from build123d import *

# Parameters (mm, degrees)
SKETCH1_W           = 19.05
SKETCH1_H           = 19.05
SKETCH1_R           = 4.8895
BOSS_EXTRUDE1_DEPTH = 3.175
SKETCH3_W           = 19.05
SKETCH3_H           = 19.05
SKETCH3_R           = 3.3782
BOSS_EXTRUDE2_DEPTH = 3.175
SKETCH4_W           = 19.05
SKETCH4_H           = 19.05
BOSS_EXTRUDE3_DEPTH = 3.175
FILLET1_R           = 3.175


with BuildPart() as part:
    # Sketch1 → Boss-Extrude1 (new body)
    with BuildSketch(Plane(origin=(0, 0, 0), x_dir=(1, 0, 0), z_dir=(0, 1, 0))):
        Rectangle(SKETCH1_W, SKETCH1_H)
        Circle(SKETCH1_R, mode=Mode.SUBTRACT)
    extrude(amount=BOSS_EXTRUDE1_DEPTH)

    # Sketch3 → Boss-Extrude2 (add)
    with BuildSketch(Plane.XZ):
        Rectangle(SKETCH3_W, SKETCH3_H)
        Circle(SKETCH3_R, mode=Mode.SUBTRACT)
    extrude(amount=BOSS_EXTRUDE2_DEPTH)

    # Sketch4 → Boss-Extrude3 (add)
    with BuildSketch(Plane.XZ.offset(3.175)):
        Rectangle(SKETCH4_W, SKETCH4_H)
    extrude(amount=BOSS_EXTRUDE3_DEPTH)

    # Fillet1
    fillet1_edges = [part.edges().sort_by_distance(p)[0] for p in [
        (-9.525, 3.175, 0),
        (0, 3.175, 9.525),
        (9.525, 3.175, 0),
        (0, 3.175, -9.525),
        (9.525, -1.5875, 9.525),
        (-9.525, -1.5875, 9.525),
        (-9.525, -1.5875, -9.525),
        (9.525, -1.5875, -9.525),
    ]]
    fillet(fillet1_edges, radius=FILLET1_R)


solid = part.part
CAD build for the part. Positions are in the model's coordinates, mm. A direction names the side the tool comes from. Round coordinates to 2 decimals unless told otherwise and drop trailing zeros. Write each loop counter-clockwise with the first axis right and the second up, starting at its lowest first coordinate (ties: lowest second). Pieces come first, ordered by that corner, then holes. Notation, with made-up numbers: (82.25, -12.5) -> (135.25, -12.5) arc R16 cw to (135.25, 16.5) -> close; hole circle Ø8 at (84.25, -14). An arc over 180 degrees is marked (long way). Answer as a JSON object with one key per item and string values.
(1) Band-saw the part on D-D, the plane y = -3.5. List the corners of the cut face in (x, z) (3 decimals), then the cut area to 3 significant figures.
Reported:
{"outline": "(-9.525, -6.35) arc R3.175 ccw to (-6.35, -9.525) -> (6.35, -9.525) arc R3.175 ccw to (9.525, -6.35) -> (9.525, 6.35) arc R3.175 ccw to (6.35, 9.525) -> (-6.35, 9.525) arc R3.175 ccw to (-9.525, 6.35) -> close", "area": "354 mm^2"}
(2) Which spindle directions (+Z, -Z, +X, -X, +Y, -Y) get a long thin tool onto all of the face, cutting with end or side? Do faces 4 (the face through (-8.62, -3.13, 8.57)), 5 (the face through (-1.06, 1.565, 4.773)). Say none if no direction does.
Reported:
{"face 4": "+Z, -X, +Y, -Y", "face 5": "+Y"}
(3) Probe probe 1 along Z at (x, y) = (0, -2) (3 decimals); probe 2 along Y at (x, z) = (1.5, 1) (3 decimals); probe 3 along Z at (x, y) = (-2, -2.5) (3 decimals). List the from-to ranges inside material, lowest first. Write a range as [from, to].
Reported:
{"probe 1": "z = [-9.525, -3.378], [3.378, 9.525]", "probe 2": "y = [-6.35, -3.175]", "probe 3": "z = [-9.525, -2.723], [2.723, 9.525]"}
(4) Band-saw the part on A-A, the plane y = -1.25. List the corners of the cut face in (x, z) (3 decimals), then the cut area to 3 significant figures.
Reported:
{"outline": "(-9.525, -6.35) arc R3.175 ccw to (-6.35, -9.525) -> (6.35, -9.525) arc R3.175 ccw to (9.525, -6.35) -> (9.525, 6.35) arc R3.175 ccw to (6.35, 9.525) -> (-6.35, 9.525) arc R3.175 ccw to (-9.525, 6.35) -> close; hole circle Ø6.756 at (0, 0)", "area": "318 mm^2"}
(5) Two-plate mould, pull along Z, no slides. Class faces 1 (the face through (0, -3.175, 0)), 2 (the face through (8.62, 2.22, -0.09)), 3 (the face through (0.09, 2.27, 8.57)): +Z half, -Z half, draft (parallel to the pull), parting line (faces both ways), or undercut.
Reported:
{"face 1": "undercut", "face 2": "draft", "face 3": "+Z half"}
(6) Pin check, flat tips, straight feed: P1, Ø1.5, axis at y = 1, z = 0, coming from the +X side; P2, Ø4, axis at x = 1, y = 0.5, coming from the -Z side (3 decimals); P3, Ø2, axis at x = 0.5, z = 0.5, coming from the +Y side (3 decimals); P4, Ø8, axis at x = 0, z = 0.5, coming from the +Y side. Stop position of each tip, or through.
Reported:
{"P1": "stops at x = 9.52", "P2": "stops at z = -9.525", "P3": "stops at y = -3.175", "P4": "stops at y = 0"}
